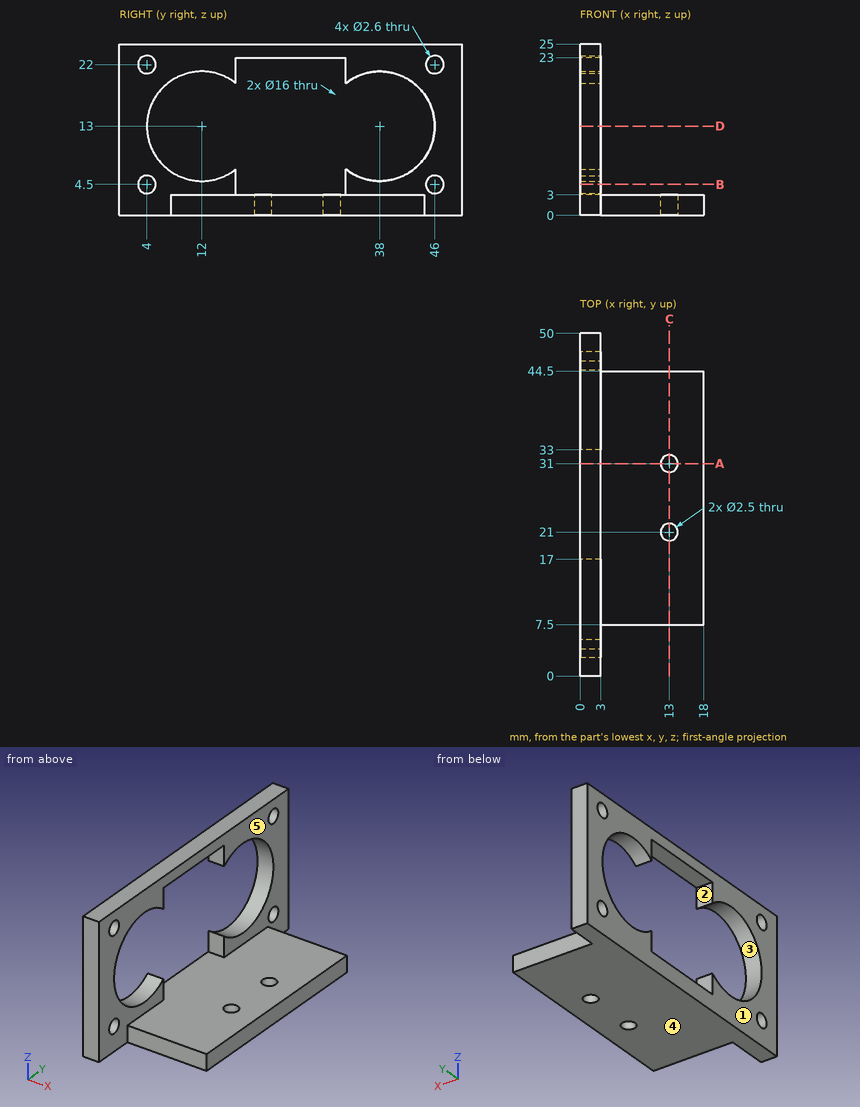
Verification items for this drawing (mm, ordinates from the low corner). A direction names the side the tool comes from. Coordinates: 2 decimals unless noted, no trailing zeros. Order: outer loops, then holes, each group sorted by start corner. A loop starts at its lowest first (then second) coordinate and runs counter-clockwise, first axis right, second up. Notation, with made-up numbers: (2, 59.25) - (18, 59.25) arc R25 cw to (18, 93.25) - close; hole circle Ø7 at (9, 14.25). An arc over 180 degrees is marked (long way). Use one line per item in the form item = value.
1. Gauge pin test, flat ends, axial feed: pin 1 (0.9 mm diameter, centred on x = 13, z = 1, fed in from -Y); pin 2 (3 mm diameter, centred on x = 7.5, z = 3.5, fed in from +Y); pin 3 (3 mm diameter, centred on x = 13, y = 21, fed in from -Z); pin 4 (1.5 mm diameter, centred on x = 4, z = 17, fed in from +Y). Record the tip position at first contact, or that the pin passes through.
Here are the results:
pin_1 = 7.5
pin_2 = 44.5
pin_3 = 0
pin_4 = through
2. Section check C-C (x = 13). Record the boundary of the cut face in (y, z), then the cut area to 3 significant figures.
Here are the results:
outline = (7.5, 0) - (19.75, 0) - (19.75, 3) - (7.5, 3) - close; (22.25, 0) - (29.75, 0) - (29.75, 3) - (22.25, 3) - close; (32.25, 0) - (44.5, 0) - (44.5, 3) - (32.25, 3) - close
area = 96.0 mm²
3. Section check A-A (y = 31). Record the boundary of the cut face in (x, z), then the cut area to 3 significant figures.
Here are the results:
outline = (0, 0) - (11.75, 0) - (11.75, 3) - (0, 3) - close; (0, 23) - (3, 23) - (3, 25) - (0, 25) - close; (14.25, 0) - (18, 0) - (18, 3) - (14.25, 3) - close
area = 52.5 mm²
4. Section check B-B (z = 4.5). Record the boundary of the cut face in (x, y), then the cut area to 3 significant figures.
Here are the results:
outline = (0, 0) - (3, 0) - (3, 2.7) - (0, 2.7) - close; (0, 5.3) - (3, 5.3) - (3, 17) - (0, 17) - close; (0, 33) - (3, 33) - (3, 44.7) - (0, 44.7) - close; (0, 47.3) - (3, 47.3) - (3, 50) - (0, 50) - close
area = 86.4 mm²
5. Access from +Z, -Z, +X, -X, +Y, -Y to the whole of each face (thin tool, end or side, straight path). Record for the marked faces 1 and 2.
Here are the results:
face_1 = +Z, -Z, -X, +Y, -Y
face_2 = +X, -X
6. Scan lines: line 1 (Z direction, x = 1, y = 3.5); line 2 (Y direction, x = 1.9, z = 13); line 3 (X direction, y = 46, z = 16.5). Record each from-to range of solid material in increasing order.
Here are the results:
line_1 = 0 to 3.3, 5.7 to 20.8, 23.2 to 25
line_2 = 0 to 4, 46 to 50
line_3 = 0 to 3
7. Section check D-D (z = 13). Record the boundary of the cut face in (x, y), then the cut area to 3 significant figures.
Here are the results:
outline = (0, 0) - (3, 0) - (3, 4) - (0, 4) - close; (0, 46) - (3, 46) - (3, 50) - (0, 50) - close
area = 24.0 mm²
8. Draft check along Z on the marked faces 3, 4 and 5. Enter one of: pulls with the +Z half, pulls with the -Z half, needs draft (parallel to the pull), parting line crosses it, or undercut.
Here are the results:
face_3 = undercut
face_4 = pulls with the -Z half
face_5 = needs draft
